```python
from build123d import *

# Parameters (mm, degrees)
RESSALTO_EXTRUS_O1_DEPTH = 4.5


with BuildPart() as part:
    # Esboço1 → Ressalto-extrusão1 (new body, symmetric)
    with BuildSketch(Plane.XY):
        with BuildLine():
            ThreePointArc((203.94484, -24.4), (228.34484, 0), (203.94484, 24.4))
            Line((203.94484, 24.4), (0, 24.4))
            ThreePointArc((0, 24.4), (-24.4, 0), (0, -24.4))
            Line((0, -24.4), (203.94484, -24.4))
        make_face()
        with BuildLine():
            ThreePointArc((0, -21.4), (-21.4, 0), (0, 21.4))
            Line((0, 21.4), (203.94484, 21.4))
            ThreePointArc((203.94484, 21.4), (225.34484, 0), (203.94484, -21.4))
            Line((203.94484, -21.4), (0, -21.4))
        make_face(mode=Mode.SUBTRACT)
    extrude(amount=RESSALTO_EXTRUS_O1_DEPTH, both=True)


solid = part.part
```
Check sheet for the modelled part. Datum: model origin and axes. Units: mm. A direction names the side the tool comes from. Round coordinates to 2 decimals unless told otherwise and drop trailing zeros. Order: outer loops, then holes, each group sorted by start corner. A loop starts at its lowest first (then second) coordinate and runs counter-clockwise, first axis right, second up. Notation, with made-up numbers: (-9.75, 42) -> (20.25, 42) arc R14 cw to (20.25, 49) -> close; hole circle Ø8 at (82, -20.5). An arc over 180 degrees is marked (long way). One line per item, written item: value. Start each with the question number.
Q1. Cross-section at C-C (y = 0). Record the boundary of the cut face in (x, z).
Q2. Mould release check, pull along X, two halves, no side actions. Record for faces 3 (the face through (101, -22, 4.5)), 4 (the face through (228.34, -0.54, 0.06)), 5 (the face through (103, -21.4, 0)): pulls with the +X half, pulls with the -X half, needs draft (parallel to the pull), parting line crosses it, or undercut.
Q3. Thickness scan on line 1 (Y direction, x = 94.5, z = -0.5); line 2 (X direction, y = 8, z = 1.5); line 3 (X direction, y = 11.5, z = 0.75). Record the ranges inside material, lowest first.
Q4. Gauge pin test, flat ends, axial feed: pin 1 Ø1 at (y, z) = (1, -2.5) entering from +X; pin 2 Ø1 at (y, z) = (-4.5, -2) entering from -X; pin 3 Ø2 at (y, z) = (-19, -1.5) entering from +X. Record the tip position at first contact, or that the pin passes through.
Q5. Cross-section at B-B (z = 0.25). Record the boundary of the cut face in (x, y), and give its area (3 significant figures).
Q6. Cross-section at A-A (x = 195). Record the boundary of the cut face in (y, z), and give its area (3 significant figures).
Q7. Set-up check for faces 1 (the face through (-24.394, 0.537, 0.063)), 2 (the face through (-21.395, -0.471, 0.063)): record each of +Z, -Z, +X, -X, +Y, -Y from which the full face is reachable in a straight line by a thin tool's end or side.
Completed:
1. outline: (-24.4, -4.5) -> (-21.4, -4.5) -> (-21.4, 4.5) -> (-24.4, 4.5) -> close; (225.34, -4.5) -> (228.34, -4.5) -> (228.34, 4.5) -> (225.34, 4.5) -> close
2. face 3: needs draft
2. face 4: pulls with the +X half
2. face 5: undercut
3. line 1: y = -24.4 to -21.4, 21.4 to 24.4
3. line 2: x = -23.05 to -19.85, 223.79 to 227
3. line 3: x = -21.52 to -18.05, 221.99 to 225.46
4. pin 1: stops at x = 228.34
4. pin 2: stops at x = -24.07
4. pin 3: stops at x = 220.42
5. outline: (0, -24.4) -> (203.94, -24.4) arc R24.4 ccw to (203.94, 24.4) -> (0, 24.4) arc R24.4 ccw to start; hole (0, -21.4) -> (203.94, -21.4) arc R21.4 ccw to (203.94, 21.4) -> (0, 21.4) arc R21.4 ccw to start
5. area: 1,660 mm²
6. outline: (-24.4, -4.5) -> (-21.4, -4.5) -> (-21.4, 4.5) -> (-24.4, 4.5) -> close; (21.4, -4.5) -> (24.4, -4.5) -> (24.4, 4.5) -> (21.4, 4.5) -> close
6. area: 54.0 mm²
7. face 1: +Z, -Z, -X
7. face 2: +Z, -Z
